from build123d import *
from build123d.topology import SkipClean

# Parameters (mm, degrees)
BOSS_EXTRUDE1_DEPTH      = 19.75
FILLET1_RADIUS           = 9.875
FILLET1_LENGTH           = 48
SKETCH2_R                = 7.55
CUT_EXTRUDE1_DEPTH       = 70.718810231
BOSS_EXTRUDE2_START      = -23
SKETCH3_R                = 6.2
BOSS_EXTRUDE2_DEPTH      = 23
SKETCH4_R                = 4.2
CUT_EXTRUDE2_DEPTH       = 56.624185387
SKETCH5_W                = 7
SKETCH5_H                = 6.5
CUT_EXTRUDE3_DEPTH       = 56.624185387
BOSS_EXTRUDE3_DEPTH      = 4
CUT_EXTRUDE4_REACH       = 60.092
SKETCH7_W                = 6.5
SKETCH7_H                = 7.7
BOSS_EXTRUDE4_DEPTH      = 5.5
SKETCH9_W                = 6.5
SKETCH9_H                = 7.7
CUT_EXTRUDE5_DEPTH       = 14
BOSS_EXTRUDE5_DEPTH      = 4
BOSS_EXTRUDE6_REACH      = 53.302
SKETCH11_R               = 4.25
CUT_EXTRUDE7_DEPTH       = 55.36094646
CUT_EXTRUDE7_DEPTH_BACK  = 5
SKETCH13_W               = 8.5
SKETCH13_H               = 5.1
CUT_EXTRUDE8_DEPTH       = 2.5
CUT_EXTRUDE6_REACH       = 56.361
SKETCH12_R               = 2.6
BOSS_EXTRUDE7_REACH      = 45.123
BOSS_EXTRUDE7_END_RADIUS = 9.875
SKETCH17_W               = 2.341574484
SKETCH17_H               = 1
CUT_EXTRUDE9_DEPTH       = 70.718810231
BOSS_EXTRUDE8_START      = -1
BOSS_EXTRUDE8_DEPTH      = 0.5
LPATTERN1_COUNT          = 7
LPATTERN1_PITCH          = 7.75
SKETCH19_R               = 4.5
CUT_EXTRUDE10_DEPTH      = 2.5


with BuildPart() as part:
    # Sketch1 → Boss-Extrude1 (new body)
    with BuildSketch(Plane(origin=(0, 0, 0), x_dir=(1, 0, 0), z_dir=(0, 1, 0))):
        with BuildLine():
            Line((16.074136013, -31.9), (6.75, -31.9))
            Line((6.75, -31.9), (6.75, -38.4))
            Line((6.75, -38.4), (8, -38.4))
            Line((8, -38.4), (8, -42.4))
            Line((8, -42.4), (-8, -42.4))
            Line((-8, -42.4), (-8, -38.4))
            Line((-8, -38.4), (-6.75, -38.4))
            Line((-6.75, -38.4), (-6.75, -31.9))
            Line((-6.75, -31.9), (-16.074136013, -31.9))
            ThreePointArc((-16.074136013, -31.9), (-26.076909961, -33.082331313), (-24, -23.226376819))
            Line((-24, -23.226376819), (-24, 0))
            Line((-24, 0), (24, 0))
            Line((24, 0), (24, -23.226376819))
            ThreePointArc((24, -23.226376819), (26.076909961, -33.082331313), (16.074136013, -31.9))
        make_face()
    extrude(amount=BOSS_EXTRUDE1_DEPTH)

    # Fillet1: full round fillet: the end face becomes a half cylinder, R = half its width
    fillet1_face = Plane((0, 9.875, 0), x_dir=(1, 0, 0), z_dir=(0, 0, -1))  # on the end face: x along it, z out of the body
    fillet1_slab = fillet1_face.offset(-FILLET1_RADIUS / 2) * Box(FILLET1_LENGTH, 2 * FILLET1_RADIUS, FILLET1_RADIUS, mode=Mode.PRIVATE)  # the body's end, R deep
    fillet1_round = Plane((0, 9.875, 9.875), x_dir=(0, 0, -1), z_dir=(1, 0, 0)) * Cylinder(FILLET1_RADIUS, FILLET1_LENGTH, mode=Mode.PRIVATE)  # its axis R under the face
    add(fillet1_slab - fillet1_round, mode=Mode.SUBTRACT)

    # Sketch2 → Cut-Extrude1 (cut, through all)
    with BuildSketch(Plane(origin=(24, 0, 0), x_dir=(0, 0, -1), z_dir=(1, 0, 0))):
        with Locations((-9.875, 9.875)):
            Circle(SKETCH2_R)
    extrude(amount=-CUT_EXTRUDE1_DEPTH, mode=Mode.SUBTRACT)

    # Sketch3 → Boss-Extrude2 (add)
    with SkipClean():  # the faces are left unmerged after this step: merging them gives an invalid solid
        with BuildSketch(Plane(origin=(0, 19.75, 0), x_dir=(1, 0, 0), z_dir=(0, 1, 0)).offset(BOSS_EXTRUDE2_START)):
            with Locations(Location((21.5, -28.9, 0), (0, 0, 66.220005269))):
                Circle(SKETCH3_R)
            with Locations(Location((-21.5, -28.9, 0), (0, 0, 113.779994731))):
                Circle(SKETCH3_R)
        extrude(amount=BOSS_EXTRUDE2_DEPTH)

    # Sketch4 → Cut-Extrude2 (cut, through all)
    with SkipClean():  # the faces are left unmerged after this step: merging them gives an invalid solid
        with BuildSketch(Plane(origin=(0, 19.75, 0), x_dir=(1, 0, 0), z_dir=(0, 1, 0))):
            with Locations(Location((-21.5, -28.9, 0), (0, 0, 270))):
                Circle(SKETCH4_R)
            with Locations(Location((21.5, -28.9, 0), (0, 0, 270))):
                Circle(SKETCH4_R)
        extrude(amount=-CUT_EXTRUDE2_DEPTH, mode=Mode.SUBTRACT)

    # Sketch5 → Cut-Extrude3 (cut, through all)
    with BuildSketch(Plane(origin=(0, 19.75, 0), x_dir=(1, 0, 0), z_dir=(0, 1, 0))):
        with Locations((0, -23.15)):
            Rectangle(SKETCH5_W, SKETCH5_H)
        with Locations((0, -35.15)):
            Rectangle(SKETCH5_W, SKETCH5_H)
        with BuildLine():
            Line((17, -19.9), (7, -19.9))
            Line((7, -19.9), (7, -26.4))
            Line((7, -26.4), (8, -26.4))
            Line((8, -26.4), (8, -27.9))
            Line((8, -27.9), (15.381176584, -27.9))
            ThreePointArc((15.381176584, -27.9), (15.945284357, -26.145887779), (17, -24.635026378))
            Line((17, -24.635026378), (17, -19.9))
        make_face()
        with BuildLine():
            Line((-7, -19.9), (-17, -19.9))
            Line((-17, -19.9), (-17, -24.635026378))
            ThreePointArc((-17, -24.635026378), (-15.945284357, -26.145887779), (-15.381176584, -27.9))
            Line((-15.381176584, -27.9), (-8, -27.9))
            Line((-8, -27.9), (-8, -26.4))
            Line((-8, -26.4), (-7, -26.4))
            Line((-7, -26.4), (-7, -19.9))
        make_face()
    extrude(amount=-CUT_EXTRUDE3_DEPTH, mode=Mode.SUBTRACT)

    # Sketch6 → Boss-Extrude3 (add)
    with BuildSketch(Plane.XY.offset(42.4)):
        with BuildLine():
            Line((-8, 0), (-8, -1.25))
            ThreePointArc((-8, -1.25), (0, -9.25), (8, -1.25))
            Line((8, -1.25), (8, 0))
            Line((8, 0), (-8, 0))
        make_face()
    extrude(amount=-BOSS_EXTRUDE3_DEPTH)

    # Cut-Extrude4: up to this face of the body (flat: up to its plane)
    cut_extrude4_end = Plane(part.part.faces().sort_by_distance((-6.75, 9.875, 35.15))[0])
    # Sketch7 → Cut-Extrude4 (cut, up to the picked face)
    with BuildSketch(Plane(origin=(6.75, 0, 0), x_dir=(0, 0, -1), z_dir=(1, 0, 0)), mode=Mode.PRIVATE) as cut_extrude4_sk1:
        with Locations((-35.15, 3.85)):
            Rectangle(SKETCH7_W, SKETCH7_H)
    cut_extrude4_tool1 = split(extrude(cut_extrude4_sk1.sketch, amount=-CUT_EXTRUDE4_REACH, mode=Mode.PRIVATE), bisect_by=cut_extrude4_end, keep=Keep.BOTH, mode=Mode.PRIVATE)
    add(cut_extrude4_tool1.solids().sort_by(Axis((6.75, 3.85, 35.15), (-1, 0, 0)))[0], mode=Mode.SUBTRACT)

    # Sketch8 → Boss-Extrude4 (add)
    with BuildSketch(Plane.XY.offset(31.9)):
        with BuildLine():
            Line((-8, -1.25), (-8, 0))
            Line((-8, 0), (8, 0))
            Line((8, 0), (8, -1.25))
            ThreePointArc((8, -1.25), (0, -9.25), (-8, -1.25))
        make_face()
    extrude(amount=-BOSS_EXTRUDE4_DEPTH)

    # Sketch9 → Cut-Extrude5 (cut)
    with BuildSketch(Plane(origin=(7, 0, 0), x_dir=(0, 0, -1), z_dir=(1, 0, 0))):
        with Locations((-23.15, 3.85)):
            Rectangle(SKETCH9_W, SKETCH9_H)
    extrude(amount=-CUT_EXTRUDE5_DEPTH, mode=Mode.SUBTRACT)

    # Sketch10 → Boss-Extrude5 (add)
    with BuildSketch(Plane.XY.offset(19.9)):
        with BuildLine():
            Line((-8, -1.25), (-8, 0))
            Line((-8, 0), (8, 0))
            Line((8, 0), (8, -1.25))
            ThreePointArc((8, -1.25), (0, -9.25), (-8, -1.25))
        make_face()
    extrude(amount=-BOSS_EXTRUDE5_DEPTH)

    # Boss-Extrude6: up to this face of the body (flat: up to its plane)
    boss_extrude6_end = Plane(part.part.faces().sort_by_distance((0, 13.725, 19.9))[0])
    # Sketch11 → Boss-Extrude6 (add, up to the picked face)
    with BuildSketch(Plane(origin=(0, 0, 38.4), x_dir=(-1, 0, 0), z_dir=(0, 0, -1)), mode=Mode.PRIVATE) as boss_extrude6_sk1:
        with Locations(Location((0, -1.25, 0), (0, 0, 180))):
            Circle(SKETCH11_R)
    boss_extrude6_tool1 = split(extrude(boss_extrude6_sk1.sketch, amount=BOSS_EXTRUDE6_REACH, mode=Mode.PRIVATE), bisect_by=boss_extrude6_end, keep=Keep.BOTH, mode=Mode.PRIVATE)
    add(boss_extrude6_tool1.solids().sort_by(Axis((0, -1.25, 38.4), (0, 0, -1)))[0])

    # Sketch13 → Cut-Extrude7 (cut, two sides: drawn at the far end of the back side and taken through both)
    with BuildSketch(Plane.XZ.offset(-CUT_EXTRUDE7_DEPTH_BACK)):
        with Locations((0, 35.15)):
            Rectangle(SKETCH13_W, SKETCH13_H)
        with Locations((0, 23.15)):
            Rectangle(SKETCH13_W, SKETCH13_H)
    extrude(amount=CUT_EXTRUDE7_DEPTH + CUT_EXTRUDE7_DEPTH_BACK, mode=Mode.SUBTRACT)

    # Sketch15 → Cut-Extrude8 (cut, symmetric)
    with BuildSketch(Plane(origin=(0, 0, 0), x_dir=(0, 0, -1), z_dir=(1, 0, 0))):
        with BuildLine():
            Line((-15.9, 0), (-15.9, 2.050998466))
            ThreePointArc((-15.9, 2.050998466), (-13.05726412, 0.526801239), (-9.875, 0))
            Line((-9.875, 0), (-15.9, 0))
        make_face()
    extrude(amount=CUT_EXTRUDE8_DEPTH, both=True, mode=Mode.SUBTRACT)

    # Cut-Extrude6: up to this face of the body (flat: up to its plane)
    cut_extrude6_end = Plane(part.part.faces().sort_by_distance((0, -3.978206263, 15.9))[0])
    # Sketch12 → Cut-Extrude6 (cut, up to the picked face)
    with BuildSketch(Plane.XY.offset(42.4), mode=Mode.PRIVATE) as cut_extrude6_sk1:
        with Locations((0, -1.25)):
            Circle(SKETCH12_R)
    cut_extrude6_tool1 = split(extrude(cut_extrude6_sk1.sketch, amount=-CUT_EXTRUDE6_REACH, mode=Mode.PRIVATE), bisect_by=cut_extrude6_end, keep=Keep.BOTH, mode=Mode.PRIVATE)
    add(cut_extrude6_tool1.solids().sort_by(Axis((0, -1.25, 42.4), (0, 0, -1)))[0], mode=Mode.SUBTRACT)

    # Boss-Extrude7: up to this cylinder (the profile starts outside it)
    boss_extrude7_end = Plane(origin=(2.389901, 9.875, 9.875), z_dir=(1, 0, 0)) * Cylinder(BOSS_EXTRUDE7_END_RADIUS, 110.996, mode=Mode.PRIVATE)
    # Sketch16 → Boss-Extrude7 (add, up to the surface)
    with BuildSketch(Plane(origin=(0, 0, 15.9), x_dir=(-1, 0, 0), z_dir=(0, 0, -1)), mode=Mode.PRIVATE) as boss_extrude7_sk1:
        with BuildLine():
            Line((-2.279802623, 0), (-2.5, 0))
            Line((-2.5, 0), (-2.5, 1.800187721))
            Line((-2.5, 1.800187721), (2.5, 1.800187721))
            Line((2.5, 1.800187721), (2.5, 0))
            Line((2.5, 0), (2.279802623, 0))
            ThreePointArc((2.279802623, 0), (0, 1.35), (-2.279802623, 0))
        make_face()
    boss_extrude7_tool1 = extrude(boss_extrude7_sk1.sketch, amount=BOSS_EXTRUDE7_REACH, mode=Mode.PRIVATE) - boss_extrude7_end
    add(boss_extrude7_tool1.solids().sort_by_distance((2.389901, 0.053142, 15.9))[0])

    # Sketch17 → Cut-Extrude9 (cut, through all)
    with BuildSketch(Plane.ZY.offset(24)):
        with Locations((1.170787242, 9.875)):
            Rectangle(SKETCH17_W, SKETCH17_H)
    extrude(amount=-CUT_EXTRUDE9_DEPTH, mode=Mode.SUBTRACT)

    # Sketch18 → Boss-Extrude8 (add)
    with BuildSketch(Plane.ZY.offset(24).offset(BOSS_EXTRUDE8_START)):
        with BuildLine():
            Line((0.012666351, 10.375), (2.341574484, 10.375))
            ThreePointArc((2.341574484, 10.375), (2.325, 9.875), (2.341574484, 9.375))
            Line((2.341574484, 9.375), (0.012666351, 9.375))
            ThreePointArc((0.012666351, 9.375), (0, 9.875), (0.012666351, 10.375))
        make_face()
    boss_extrude8 = extrude(amount=BOSS_EXTRUDE8_DEPTH)

    # LPattern1: Boss-Extrude8 ×7
    with Locations(*[(i * LPATTERN1_PITCH, 0, 0) for i in range(1, LPATTERN1_COUNT)]):
        add(boss_extrude8)

    # Sketch19 → Cut-Extrude10 (cut)
    with BuildSketch(Plane.XY.offset(42.4)):
        with Locations((0, -1.25)):
            Circle(SKETCH19_R)
    extrude(amount=-CUT_EXTRUDE10_DEPTH, mode=Mode.SUBTRACT)


solid = part.part
Work out the finished part from the listing and answer in its coordinate system (mm). A direction names the side the tool comes from. Round coordinates to 2 decimals unless told otherwise and drop trailing zeros. Write each loop counter-clockwise with the first axis right and the second up, starting at its lowest first coordinate (ties: lowest second). Pieces come first, ordered by that corner, then holes. Notation, with made-up numbers: (18, -28) - (33, -28) arc R34 cw to (33, 9) - close; hole circle Ø10 at (71, -39.5). An arc over 180 degrees is marked (long way). Answer in a Markdown table with one row per item. Add a question column.
1. A cutting plane is placed at D-D, the plane z = 36.5. Determine the outline of the cut face in (x, y).
2. For faces 1 (the flat face through (0, 5, 38.4)), 2 (the cylindrical face through (-0.338, 1.328, 38.815)), 3 (the flat face through (-8, 9, 40)), 4 (the flat face through (-8, -1, 18)), 5 (the flat face through (-7, 14, 23)), determine the directions among +Z, -Z, +X, -X, +Y, -Y from which every point of the face is accessible in a straight line to the end or side of a thin tool.
3. A cutting plane is placed at B-B, the plane x = 21.5. Determine the outline of the cut face in (y, z) (3 decimals).
4. A cutting plane is placed at C-C, the plane y = -7. Determine the outline of the cut face in (x, z), and give its area (3 significant figures).
5. Find the intervals of material crossed by line 1 along Z through (x, y) = (3, -4.5), in increasing order. Write a range as from..to.
6. The mould has two halves that part along Y. Classify faces 6 (the flat face through (-12, 0, 30)), 7 (the flat face through (-12, 10.375, 1)), 8 (the flat face through (8, 7.7, 27.5)): +Y half, -Y half, draft (parallel to the pull), parting line (faces both ways), or undercut.
7. Given pin 1 (1 mm diameter, centred on x = 8.5, y = 13.5, fed in from -Z); pin 2 (0.6 mm diameter, centred on x = 23.5, z = 1, fed in from -Y); pin 3 (3 mm diameter, centred on x = 4.5, z = 22.5, fed in from -Y), each flat-ended and moving along its own axis, determine where each tip first touches the part or whether it passes through.
Worked out:
| question | item | result |
|---|---|---|
| 1 | outline | (-6.75, 7.7) - (-3.5, 7.7) - (-3.5, 19.75) - (-6.75, 19.75) - close; (3.5, 7.7) - (6.75, 7.7) - (6.75, 19.75) - (3.5, 19.75) - close |
| 2 | face 1 | none |
| 2 | face 2 | +Z |
| 2 | face 3 | +Z, -X, +Y, -Y |
| 2 | face 4 | +Z, -Z, -X, -Y |
| 2 | face 5 | +Y, -Y |
| 3 | outline | (-3.25, 22.7) - (0, 22.7) - (0, 9.875) arc R9.875 ccw to (9.375, 0.013) - (9.375, 2.342) arc R7.55 cw (long way) to (10.375, 2.342) - (10.375, 0.013) arc R9.875 ccw to (19.75, 9.875) - (19.75, 24.7) - (-3.25, 24.7) - close; (-3.25, 33.1) - (19.75, 33.1) - (19.75, 35.1) - (-3.25, 35.1) - close |
| 4 | outline | (-5.56, 15.9) - (5.56, 15.9) - (5.56, 19.9) - (-5.56, 19.9) - close; (-5.56, 26.4) - (5.56, 26.4) - (5.56, 31.9) - (-5.56, 31.9) - close; (-5.56, 38.4) - (5.56, 38.4) - (5.56, 42.4) - (-5.56, 42.4) - close |
| 4 | area | 150 mm^2 |
| 5 | line 1 | 15.9..19.9, 26.4..31.9, 38.4..39.9 |
| 6 | face 6 | -Y half |
| 6 | face 7 | undercut |
| 6 | face 8 | draft |
| 7 | pin 1 | z = 0.51 |
| 7 | pin 2 | y = 4.98 |
| 7 | pin 3 | y = 7.7 |
